The listing builds one solid part. Answer for the finished solid, in the listing's coordinates (mm). Face numbers are marked on the shaded views. A direction names the side the tool comes from. Give positions to 0.01 mm unless a question says otherwise; leave off trailing zeros. Order: outer loops, then holes, each group sorted by start corner. A loop starts at its lowest first (then second) coordinate and runs counter-clockwise, first axis right, second up. Notation, with made-up numbers: (-21, 79.5) -> (29, 79.5) arc R6 cw to (29, 84.5) -> close; hole circle Ø4 at (29, 45.5). An arc over 180 degrees is marked (long way). Answer as a JSON object with one key per item and string values. Group by question number.
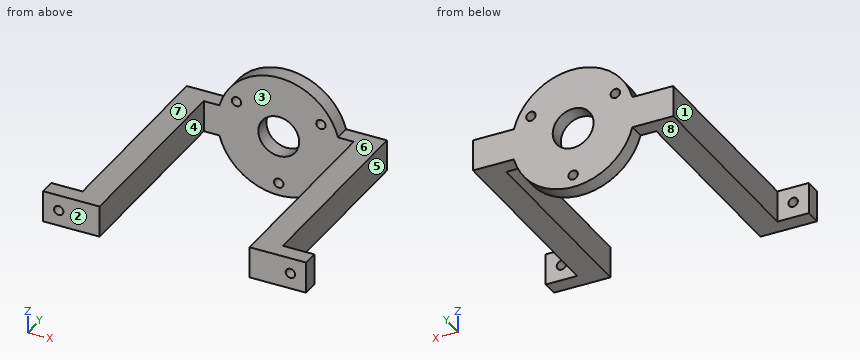
```python
from build123d import *

# Parameters (mm, degrees)
SKETCH1_R                 = 6.5
BOSS_EXTRUDE1_DEPTH       = 5
SKETCH2_W                 = 8
SKETCH2_H                 = 10
BOSS_EXTRUDE2_DEPTH       = 64
SKETCH5_W                 = 10
SKETCH5_H                 = 5
BOSS_EXTRUDE3_DEPTH       = 10
SKETCH6_W                 = 10
SKETCH6_H                 = 5
BOSS_EXTRUDE4_DEPTH       = 10
F_3_0MM_DOWEL_HOLE1_D     = 3
F_3_0MM_DOWEL_HOLE1_DEPTH = 23
F_3_0MM_DOWEL_HOLE1_TIP   = 0.901290929
F_3_0MM_DOWEL_HOLE2_D     = 3


with BuildPart() as part:
    # Sketch1 → Boss-Extrude1 (new body)
    with BuildSketch(Plane(origin=(0, 0, 0), x_dir=(1, 0, 0), z_dir=(0, 1, 0))):
        with BuildLine():
            Line((-31.848076825, -5), (-18.848076825, -5))
            ThreePointArc((-18.848076825, -5), (0, -19.5), (18.848076825, -5))
            Line((18.848076825, -5), (31.848076825, -5))
            Line((31.848076825, -5), (31.848076825, 5))
            Line((31.848076825, 5), (18.848076825, 5))
            ThreePointArc((18.848076825, 5), (0, 19.5), (-18.848076825, 5))
            Line((-18.848076825, 5), (-31.848076825, 5))
            Line((-31.848076825, 5), (-31.848076825, -5))
        make_face()
        Circle(SKETCH1_R, mode=Mode.SUBTRACT)
    extrude(amount=BOSS_EXTRUDE1_DEPTH)

    # Sketch2 → Boss-Extrude2 (add)
    with BuildSketch(Plane.XZ):
        with Locations((-27.848076825, 0)):
            Rectangle(SKETCH2_W, SKETCH2_H)
        with Locations((27.848076825, 0)):
            Rectangle(SKETCH2_W, SKETCH2_H)
    extrude(amount=BOSS_EXTRUDE2_DEPTH)

    # Sketch5 → Boss-Extrude3 (add)
    with BuildSketch(Plane.ZY.offset(31.848076825)):
        with Locations((0, -61.5)):
            Rectangle(SKETCH5_W, SKETCH5_H)
    extrude(amount=BOSS_EXTRUDE3_DEPTH)

    # Sketch6 → Boss-Extrude4 (add)
    with BuildSketch(Plane(origin=(31.848076825, 0, 0), x_dir=(0, 0, -1), z_dir=(1, 0, 0))):
        with Locations((0, -61.5)):
            Rectangle(SKETCH6_W, SKETCH6_H)
    extrude(amount=BOSS_EXTRUDE4_DEPTH)

    # Ø3.0mm Dowel Hole1
    with Locations(Plane(origin=(0, -59, 0), x_dir=(1, 0, 0), z_dir=(0, 1, 0))):
        with Locations((36.848076825, 0), (-36.848076825, 0)):
            Hole(F_3_0MM_DOWEL_HOLE1_D / 2, depth=F_3_0MM_DOWEL_HOLE1_DEPTH)
            with Locations((0, 0, -(F_3_0MM_DOWEL_HOLE1_DEPTH + F_3_0MM_DOWEL_HOLE1_TIP / 2))):  # 118° drill point
                Cone(0, F_3_0MM_DOWEL_HOLE1_D / 2, F_3_0MM_DOWEL_HOLE1_TIP, mode=Mode.SUBTRACT)

    # Ø3.0mm Dowel Hole2 (through all)
    with Locations(Plane(origin=(0, 5, 0), x_dir=(1, 0, 0), z_dir=(0, 1, 0))):
        with Locations((0, 15.5), (13.423393759, -7.75), (-13.423393759, -7.75)):
            Hole(F_3_0MM_DOWEL_HOLE2_D / 2)


solid = part.part
```
(1) Find the intervals of material crossed by line 1 along X through (y, z) = (-22, 0.5); line 2 along X through (y, z) = (2, 0); line 3 along Y through (x, z) = (-10, -16.5), in increasing order. Write a range as [from, to].
(2) Which of the six approach directions +Z, -Z, +X, -X, +Y, -Y give full straight-line access (tool end or side, diameter ignored) to the marked faces 4, 5, 6, 7 and 8?
(3) A cutting plane is placed at B-B (z = 0). Determine the outline of the cut face in (x, y).
(4) A cutting plane is placed at D-D (z = 7.75). Determine the outline of the cut face in (x, y), and give its area (3 significant figures).
(5) A cutting plane is placed at A-A (y = -15). Determine the outline of the cut face in (x, z).
(6) A cutting plane is placed at C-C (x = 0). Determine the outline of the cut face in (y, z).
(7) For a pull along X with two mould halves and no side action, classify the marked faces 1, 2 and 3 as +X half, -X half, draft (parallel to the pull), parting line (faces both ways), or undercut.
(8) Flat-ended cylindrical pins translate along their axes: pin 1 Ø5 at (y, z) = (-10, 4.5) entering from +X; pin 2 Ø8 at (x, z) = (-36, -1) entering from +Y; pin 3 Ø10.5 at (x, z) = (0, 0) entering from -Y; pin 4 Ø10 at (x, z) = (0, -14.5) entering from -Y. Find the tip coordinate at first contact, or state that the pin passes through.
Check sheet entries:
{
 "1": {"line 1": "x = [-31.85, -23.85], [23.85, 31.85]", "line 2": "x = [-31.85, -6.5], [6.5, 31.85]", "line 3": "y = [0, 5]"},
 "2": {"face 4": "+Z, -Z, -Y", "face 5": "+Z, -Z, +X, +Y", "face 6": "+Z, +X, +Y, -Y", "face 7": "+Z, -X, +Y, -Y", "face 8": "-Z, -X, +Y, -Y"},
 "3": {"outline": "(-41.85, -64) -> (-38.35, -64) -> (-38.35, -59) -> (-41.85, -59) -> close; (-35.35, -64) -> (-23.85, -64) -> (-23.85, 0) -> (-6.5, 0) -> (-6.5, 5) -> (-31.85, 5) -> (-31.85, -59) -> (-35.35, -59) -> close; (6.5, 0) -> (23.85, 0) -> (23.85, -64) -> (35.35, -64) -> (35.35, -59) -> (31.85, -59) -> (31.85, 5) -> (6.5, 5) -> close; (38.35, -64) -> (41.85, -64) -> (41.85, -59) -> (38.35, -59) -> close"},
 "4": {"outline": "(-17.89, 0) -> (-14.92, 0) -> (-14.92, 5) -> (-17.89, 5) -> close; (-11.92, 0) -> (11.92, 0) -> (11.92, 5) -> (-11.92, 5) -> close; (14.92, 0) -> (17.89, 0) -> (17.89, 5) -> (14.92, 5) -> close", "area": "149 mm2"},
 "5": {"outline": "(-31.85, -5) -> (-23.85, -5) -> (-23.85, 5) -> (-31.85, 5) -> close; (23.85, -5) -> (31.85, -5) -> (31.85, 5) -> (23.85, 5) -> close"},
 "6": {"outline": "(0, -19.5) -> (5, -19.5) -> (5, -17) -> (0, -17) -> close; (0, -14) -> (5, -14) -> (5, -6.5) -> (0, -6.5) -> close; (0, 6.5) -> (5, 6.5) -> (5, 19.5) -> (0, 19.5) -> close"},
 "7": {"face 1": "-X half", "face 2": "draft", "face 3": "undercut"},
 "8": {"pin 1": "stops at x = 31.85", "pin 2": "stops at y = -59", "pin 3": "passes through", "pin 4": "stops at y = 0"}
}
